Study the drawing (mm; zero at the part's minimum x, y, z) and answer. Round coordinates to 2 decimals unless told otherwise and drop trailing zeros. Order: outer loops, then holes, each group sorted by start corner. A loop starts at its lowest first (then second) coordinate and runs counter-clockwise, first axis right, second up. Notation, with made-up numbers: (25, 73.5) -> (61, 73.5) arc R21 ccw to (61, 90.5) -> close; hole circle Ø4 at (-26, -33). An arc over 180 degrees is marked (long way). Answer in a Markdown table with one row per item. Add a question column.
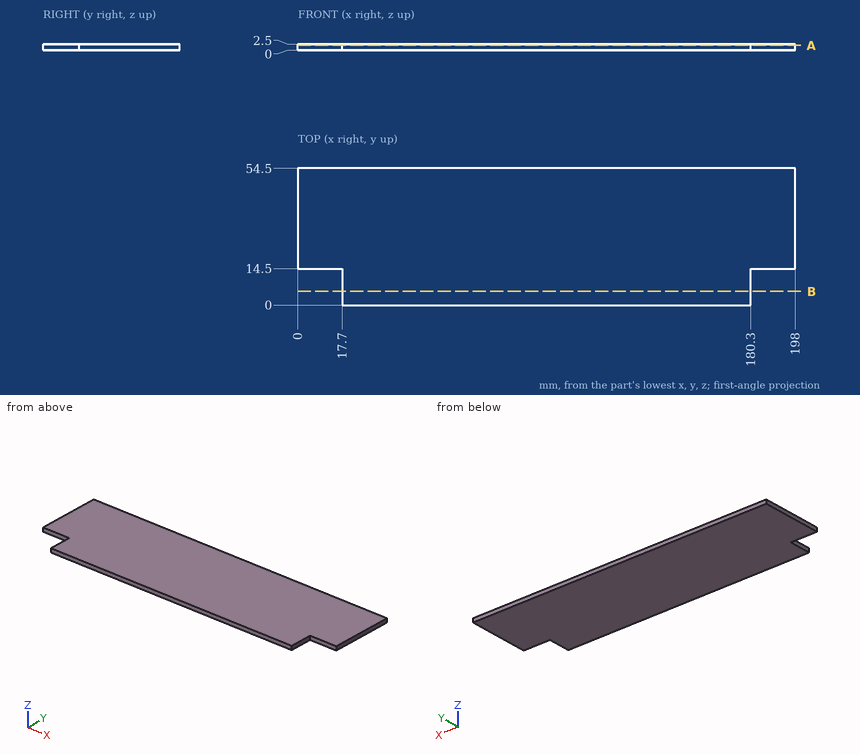
Item 1: The part is cut by section B-B, the plane y = 5.5. Give the vertices of the cut face in (x, z), and give its area (4 significant figures).
Item 2: Flat-ended cylindrical pins translate along their axes: P1, Ø0.8, axis at y = 10, z = 1.5, coming from the +X side; P2, Ø0.8, axis at y = 5.5, z = 2, coming from the -X side; P3, Ø1.2, axis at x = 6, z = 1, coming from the -Y side. Find the tip coordinate at first contact, or state that the pin passes through.
Item 3: Find the intervals of material crossed by probe 1 along X at (y, z) = (7, 1.55), in increasing order. Write a range as [from, to].
Item 4: The part is cut by section A-A, the plane z = 1.95. Give the vertices of the cut face in (x, y).
Resolved:
| question | item | result |
|---|---|---|
| 1 | outline | (17.7, 0) -> (180.3, 0) -> (180.3, 2.5) -> (17.7, 2.5) -> close |
| 1 | area | 406.5 mm2 |
| 2 | P1 | x = 180.3 |
| 2 | P2 | x = 17.7 |
| 2 | P3 | y = 14.5 |
| 3 | probe 1 | [17.7, 180.3] |
| 4 | outline | (0, 14.5) -> (17.7, 14.5) -> (17.7, 0) -> (180.3, 0) -> (180.3, 14.5) -> (198, 14.5) -> (198, 54.5) -> (0, 54.5) -> close |
